```python
from build123d import *

# Parameters (mm, degrees)
SKETCH1_W           = 66
SKETCH1_H           = 29.5
SKETCH1_W_2         = 62
SKETCH1_H_2         = 25.5
SKETCH1_R           = 1.45
BOSS_EXTRUDE1_DEPTH = 3
SKETCH1_3_W         = 66
SKETCH1_3_H         = 29.5
SKETCH1_3_W_2       = 62
SKETCH1_3_H_2       = 25.5
BOSS_EXTRUDE3_DEPTH = 6
FILLET1_R           = 2
SKETCH2_W           = 8
SKETCH2_H           = 2
CUT_EXTRUDE1_DEPTH  = 2
FILLET2_R           = 2


with BuildPart() as part:
    # Sketch1 → Boss-Extrude1 (new body)
    # profile 1 of 2: a face of its own
    with BuildSketch(Plane(origin=(0, 0, 0), x_dir=(1, 0, 0), z_dir=(0, 1, 0))):
        with Locations((27.85, 9.5)):
            Rectangle(SKETCH1_W, SKETCH1_H)
        with Locations((27.85, 9.5)):
            Rectangle(SKETCH1_W_2, SKETCH1_H_2, mode=Mode.SUBTRACT)
    # profile 2 of 2: a face of its own
    with BuildSketch(Plane(origin=(0, 0, 0), x_dir=(1, 0, 0), z_dir=(0, 1, 0))):
        with Locations((27.85, 9.5)):
            Rectangle(SKETCH1_W_2, SKETCH1_H_2)
        with Locations(Location((55.7, 19, 0), (0, 0, 270))):
            Circle(SKETCH1_R, mode=Mode.SUBTRACT)
        with Locations(Location((0, 19, 0), (0, 0, 270))):
            Circle(SKETCH1_R, mode=Mode.SUBTRACT)
        with Locations(Location((55.7, 0, 0), (0, 0, 270))):
            Circle(SKETCH1_R, mode=Mode.SUBTRACT)
        with Locations(Location((0, 0, 0), (0, 0, 270))):
            Circle(SKETCH1_R, mode=Mode.SUBTRACT)
    extrude(amount=BOSS_EXTRUDE1_DEPTH)

    # Sketch1<3> → Boss-Extrude3 (add)
    with BuildSketch(Plane(origin=(0, 0, 0), x_dir=(1, 0, 0), z_dir=(0, 1, 0))):
        with Locations((27.85, 9.5)):
            Rectangle(SKETCH1_3_W, SKETCH1_3_H)
        with Locations((27.85, 9.5)):
            Rectangle(SKETCH1_3_W_2, SKETCH1_3_H_2, mode=Mode.SUBTRACT)
    extrude(amount=BOSS_EXTRUDE3_DEPTH)

    # Fillet1
    fillet1_edges = [part.edges().sort_by_distance(p)[0] for p in [
        (-5.15, 3, -24.25),
        (60.85, 3, -24.25),
        (60.85, 3, 5.25),
        (-5.15, 3, 5.25),
    ]]
    fillet(fillet1_edges, radius=FILLET1_R)

    # Sketch2 → Cut-Extrude1 (cut)
    with BuildSketch(Plane(origin=(0, 6, 0), x_dir=(1, 0, 0), z_dir=(0, 1, 0))):
        with Locations((27.85, 23.25)):
            Rectangle(SKETCH2_W, SKETCH2_H)
    extrude(amount=-CUT_EXTRUDE1_DEPTH, mode=Mode.SUBTRACT)

    # Fillet2
    fillet2_edges = [part.edges().sort_by_distance(p)[0] for p in [
        (31.85, 6, -23.25),
        (23.85, 6, -23.25),
    ]]
    fillet(fillet2_edges, radius=FILLET2_R - 0.0001)  # a hair under: the kernel refuses the full size


solid = part.part
```
CAD build for the part. Positions are in the model's coordinates, mm. A direction names the side the tool comes from. Coordinates: 2 decimals unless noted, no trailing zeros. Write each loop counter-clockwise with the first axis right and the second up, starting at its lowest first coordinate (ties: lowest second). Pieces come first, ordered by that corner, then holes. Notation, with made-up numbers: (60, 54) -> (82, 54) arc R19 cw to (82, 81) -> close; hole circle Ø6 at (-38, 20.5). An arc over 180 degrees is marked (long way). Use CSV: the item, a comma, the result in double quotes. Start each with the question number.
Item 1: Two-plate mould, pull along Z, no slides. Class faces 1 (the cylindrical face through (-4.55, 2.96, -23.68)), 2 (the cylindrical face through (60.28, 3.04, 4.65)), 3 (the cylindrical face through (0.44, 1.48, -17.62)), 4 (the flat face through (27.4, 3.8, -22.25)): +Z half, -Z half, draft (parallel to the pull), parting line (faces both ways), or undercut.
Item 2: Band-saw the part on C-C, the plane y = 0.85. Write the cut outline in (x, z).
Item 3: Band-saw the part on A-A, the plane z = -19. Write the cut outline in (x, y).
Item 4: Wall check: probe 1 along X at (y, z) = (1.7, 0); probe 2 along Z at (x, y) = (57, 1.5); probe 3 along Z at (x, y) = (14, 5.5). Give the ranges that are in metal, low to high.
Item 5: Drop flat-ended pins along their axis: P1, Ø12, axis at x = 33.5, z = -12, coming from the +Y side; P2, Ø1, axis at x = 26.5, z = -23, coming from the +Y side. Give the stop position or say it passes through.
Item 6: Band-saw the part on B-B, the plane x = 0. Write the cut outline in (y, z).
Item 7: Tool access for faces 5 (the cylindrical face through (32.45, 5.43, -23.26)), 6 (the cylindrical face through (56.14, 1.48, -17.62)), 7 (the flat face through (-3.15, 4, -9)): list every direction of +Z, -Z, +X, -X, +Y, -Y with a clear straight run to the whole face (end or side of a thin tool).
Item 8: Band-saw the part on D-D, the plane x = 27. Write the cut outline in (y, z), plus the area to 3 significant figures.
Response values:
1,face 1,"-Z half"
1,face 2,"+Z half"
1,face 3,"undercut"
1,face 4,"undercut"
2,outline,"(-5.15, -22.25) arc R2 ccw to (-3.15, -24.25) -> (58.85, -24.25) arc R2 ccw to (60.85, -22.25) -> (60.85, 3.25) arc R2 ccw to (58.85, 5.25) -> (-3.15, 5.25) arc R2 ccw to (-5.15, 3.25) -> close; hole circle Ø2.9 at (0, -19); hole circle Ø2.9 at (0, 0); hole circle Ø2.9 at (55.7, -19); hole circle Ø2.9 at (55.7, 0)"
3,outline,"(-5.15, 0) -> (-1.45, 0) -> (-1.45, 3) -> (-3.15, 3) -> (-3.15, 6) -> (-5.15, 6) -> close; (1.45, 0) -> (54.25, 0) -> (54.25, 3) -> (1.45, 3) -> close; (57.15, 0) -> (60.85, 0) -> (60.85, 6) -> (58.85, 6) -> (58.85, 3) -> (57.15, 3) -> close"
4,probe 1,"x = -5.15 to -1.45, 1.45 to 54.25, 57.15 to 60.85"
4,probe 2,"z = -24.25 to -19.64, -18.36 to -0.64, 0.64 to 5.25"
4,probe 3,"z = -24.25 to -22.25, 3.25 to 5.25"
5,P1,"stops at y = 3"
5,P2,"stops at y = 4"
6,outline,"(0, -24.25) -> (6, -24.25) -> (6, -22.25) -> (3, -22.25) -> (3, -20.45) -> (0, -20.45) -> close; (0, -17.55) -> (3, -17.55) -> (3, -1.45) -> (0, -1.45) -> close; (0, 1.45) -> (3, 1.45) -> (3, 3.25) -> (6, 3.25) -> (6, 5.25) -> (0, 5.25) -> close"
7,face 5,"-Z, +Y"
7,face 6,"+Y, -Y"
7,face 7,"+Y"
8,outline,"(0, -24.25) -> (4, -24.25) -> (4, -22.25) -> (3, -22.25) -> (3, 3.25) -> (6, 3.25) -> (6, 5.25) -> (0, 5.25) -> close"
8,area,"96.5 mm2"
